Read the model definition and answer for the solid it produces. Units are mm, in the model's axes. A direction names the side the tool comes from. Coordinates: 2 decimals unless noted, no trailing zeros. Order: outer loops, then holes, each group sorted by start corner. A loop starts at its lowest first (then second) coordinate and runs counter-clockwise, first axis right, second up. Notation, with made-up numbers: (7, -17) - (33, -17) arc R24 ccw to (33, 11) - close; hole circle Ø6 at (79, -10). An arc over 180 degrees is marked (long way). Use one line per item in the form item = value. Start each with the question number.
from build123d import *

# Parameters (mm, degrees)
SKETCH1_R               = 15
BOSS_EXTRUDE1_DEPTH     = 35
CUT_EXTRUDE4_DEPTH      = 13
CUT_EXTRUDE4_DEPTH_BACK = 16
CUT_EXTRUDE5_DEPTH      = 1.5
SKETCH7_R               = 2.1
CUT_EXTRUDE6_DEPTH      = 2.2
CUT_EXTRUDE7_REACH      = 42.927
SKETCH8_R               = 1.7


with BuildPart() as part:
    # Sketch1 → Boss-Extrude1 (new body)
    with BuildSketch(Plane(origin=(0, 0, 0), x_dir=(1, 0, 0), z_dir=(0, 1, 0))):
        with Locations(Location((0, 0, 0), (0, 0, 270))):
            Circle(SKETCH1_R)
    extrude(amount=BOSS_EXTRUDE1_DEPTH)

    # Sketch5 → Cut-Extrude4 (cut, two sides: drawn at the far end of the back side and taken through both)
    with BuildSketch(Plane(origin=(0, 0, 0), x_dir=(0, 0, -1), z_dir=(1, 0, 0)).offset(-CUT_EXTRUDE4_DEPTH_BACK)):
        Polygon((-6, 30.7), (-6, 5), (0.5, 5), (0.5, 6), (16, 6), (16, 29.7), (0.5, 29.7), (0.5, 30.7), align=None)
    extrude(amount=CUT_EXTRUDE4_DEPTH + CUT_EXTRUDE4_DEPTH_BACK, mode=Mode.SUBTRACT)

    # Sketch6 → Cut-Extrude5 (cut)
    with BuildSketch(Plane.XZ):
        with BuildLine():
            Line((-9.697937925, 8.2), (9.697937925, 8.2))
            ThreePointArc((9.697937925, 8.2), (0, -12.7), (-9.697937925, 8.2))
        make_face()
    extrude(amount=-CUT_EXTRUDE5_DEPTH, mode=Mode.SUBTRACT)

    # Sketch7 → Cut-Extrude6 (cut)
    with BuildSketch(Plane.XZ.offset(-1.5)):
        with Locations(Location((0, -6, 0), (0, 0, 270))):
            Circle(SKETCH7_R)
    extrude(amount=-CUT_EXTRUDE6_DEPTH, mode=Mode.SUBTRACT)

    # Sketch8 → Cut-Extrude7 (cut, up to next)
    with BuildSketch(Plane(origin=(0, 35, 0), x_dir=(1, 0, 0), z_dir=(0, 1, 0)), mode=Mode.PRIVATE) as cut_extrude7_sk1:
        with Locations(Location((-10, -3, 0), (0, 0, 270))):
            Circle(SKETCH8_R)
    cut_extrude7_tool1 = extrude(cut_extrude7_sk1.sketch, amount=-CUT_EXTRUDE7_REACH, mode=Mode.PRIVATE) & part.part
    # Sketch8 → Cut-Extrude7 (cut, up to next)
    with BuildSketch(Plane(origin=(0, 35, 0), x_dir=(1, 0, 0), z_dir=(0, 1, 0)), mode=Mode.PRIVATE) as cut_extrude7_sk2:
        with Locations(Location((10, -3, 0), (0, 0, 270))):
            Circle(SKETCH8_R)
    cut_extrude7_tool2 = extrude(cut_extrude7_sk2.sketch, amount=-CUT_EXTRUDE7_REACH, mode=Mode.PRIVATE) & part.part
    add(cut_extrude7_tool1.solids().sort_by_distance((-10, 35, 3))[0], mode=Mode.SUBTRACT)
    add(cut_extrude7_tool2.solids().sort_by_distance((10, 35, 3))[0], mode=Mode.SUBTRACT)


solid = part.part
Q1. A cutting plane is placed at A-A (z = 0). Give the vertices of the cut face in (x, y).
Q2. A cutting plane is placed at C-C (y = 32.5). Give the vertices of the cut face in (x, z).
Q3. A cutting plane is placed at D-D (x = -7.75). Give the vertices of the cut face in (y, z), then the cut area to 3 significant figures.
Q4. Consider probe 1 along X at (y, z) = (0.5, 0); probe 2 along X at (y, z) = (31.65, 3); probe 3 along Z at (x, y) = (0, 0.6). Determine where each line is inside the solid, lowest interval first.
Q5. Which of the six approach directions +Z, -Z, +X, -X, +Y, -Y give full straight-line access (tool end or side, diameter ignored) to faces 1 (the cylindrical face through (0.09, 2.58, -3.9)), 2 (the flat face through (0, 35, 0)), 3 (the flat face through (-1.2, 5.5, -0.5)), 4 (the cylindrical face through (-11.5, 32.9, 3.8)), 5 (the flat face through (-1, 6, -6))?
Q6. Given P1, Ø0.5, axis at x = -5, y = 5.5, coming from the +Z side; P2, Ø2.5, axis at x = -10, z = 3, coming from the +Y side; P3, Ø1, axis at y = 8, z = 9, coming from the +X side, each flat-ended and moving along its own axis, determine where each tip first touches the part or whether it passes through.
Q7. For a pull along X with two mould halves and no side action, classify faces 6 (the flat face through (-1, 29.7, -6)), 7 (the cylindrical face through (4.506, 17.255, 14.307)), 8 (the cylindrical face through (9.35, 32.88, 4.57)) as +X half, -X half, draft (parallel to the pull), parting line (faces both ways), or undercut.
Q8. A cutting plane is placed at B-B (z = 3). Give the vertices of the cut face in (x, y).
Result sheet:
q1.outline = (-15, 0) - (-12.7, 0) - (-12.7, 1.5) - (12.7, 1.5) - (12.7, 0) - (15, 0) - (15, 35) - (-15, 35) - (-15, 30.7) - (13, 30.7) - (13, 5) - (-15, 5) - close
q2.outline = circle Ø30 at (0, 0); hole circle Ø3.4 at (-10, 3); hole circle Ø3.4 at (10, 3)
q3.outline = (0, -12.84) - (6, -12.84) - (6, -0.5) - (5, -0.5) - (5, 6) - (30.7, 6) - (30.7, -0.5) - (29.7, -0.5) - (29.7, -12.84) - (35, -12.84) - (35, 12.84) - (0, 12.84) - (0, 8.2) - (1.5, 8.2) - (1.5, -10.06) - (0, -10.06) - close
q3.area = 412 mm^2
q4.probe_1 = -15 to -12.7, 12.7 to 15
q4.probe_2 = -14.7 to -11.7, -8.3 to 8.3, 11.7 to 14.7
q4.probe_3 = -15 to -12.7, 8.2 to 15
q5.face_1 = -Y
q5.face_2 = +Z, -Z, +X, -X, +Y
q5.face_3 = -X
q5.face_4 = +Y
q5.face_5 = -Z, -X
q6.P1 = 14.23
q6.P2 = 5
q6.P3 = 12.36
q7.face_6 = draft
q7.face_7 = parting line
q7.face_8 = undercut
q8.outline = (-14.7, 0) - (-12.34, 0) - (-12.34, 1.5) - (12.34, 1.5) - (12.34, 0) - (14.7, 0) - (14.7, 35) - (11.7, 35) - (11.7, 30.7) - (13, 30.7) - (13, 5) - (-14.7, 5) - close; (-14.7, 30.7) - (-11.7, 30.7) - (-11.7, 35) - (-14.7, 35) - close; (-8.3, 30.7) - (8.3, 30.7) - (8.3, 35) - (-8.3, 35) - close
